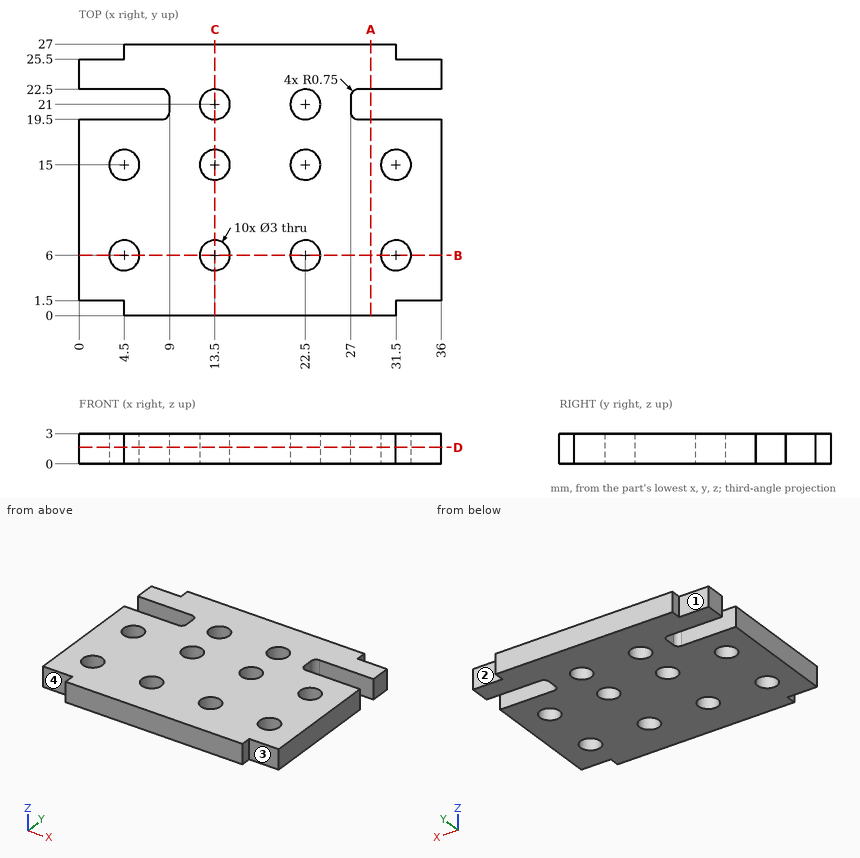
Could you check a few things on this drawing? It's one solid part, dimensions in mm from its lowest x, y, z. A direction names the side the tool comes from. Coordinates: 2 decimals unless noted, no trailing zeros. Order: outer loops, then holes, each group sorted by start corner. A loop starts at its lowest first (then second) coordinate and runs counter-clockwise, first axis right, second up. Notation, with made-up numbers: M 9.25,42 L 43.25,42 A22 ccw 43.25,48 Z; hole C 70,34 d6. An arc over 180 degrees is marked long. Use one line per item in the form item = value. Start each with the question number.
1. Suppose I cut it at A-A on x = 29. Write out the boundary of the cut face in (y, z), then the cut area to 3 significant figures.
2. Suppose I cut it at B-B on y = 6. Write out the boundary of the cut face in (x, z).
3. For pin 1 (1.5 mm diameter, centred on x = 3.5, z = 1, fed in from -Y); pin 2 (1.6 mm diameter, centred on y = 21, z = 1, fed in from -X); pin 3 (0.8 mm diameter, centred on y = 1, z = 2, fed in from -X); pin 4 (1.2 mm diameter, centred on y = 26, z = 1, fed in from -X), each with a flat end and sliding along its axis, tell me the tip position at first contact or that it passes through.
4. Suppose I cut it at D-D on z = 1.65. Count the separate pieces of the cut face and the enclosed holes in it, then the cut area to 3 significant figures.
5. Suppose I cut it at C-C on x = 13.5. Write out the boundary of the cut face in (y, z), then the cut area to 3 significant figures.
6. On a 3-axis mill with a long thin cutter (end or side, diameter ignored), from which of +Z, -Z, +X, -X, +Y, -Y can I reach the whole of each face in a straight line? I mean the marked faces 1, 2, 3 and 4. Say none if no direction works.
7. Please list where these lines run through material, in increasing order: line 1 (X direction, y = 6, z = 2.2); line 2 (Y direction, x = 13.5, z = 1.25); line 3 (X direction, y = 21, z = 2.2).
Geometry says:
q1.outline = M 0,0 L 19.5,0 L 19.5,3 L 0,3 Z; M 22.5,0 L 27,0 L 27,3 L 22.5,3 Z
q1.area = 72.0 mm^2
q2.outline = M 0,0 L 3,0 L 3,3 L 0,3 Z; M 6,0 L 12,0 L 12,3 L 6,3 Z; M 15,0 L 21,0 L 21,3 L 15,3 Z; M 24,0 L 30,0 L 30,3 L 24,3 Z; M 33,0 L 36,0 L 36,3 L 33,3 Z
q3.pin_1 = 1.5
q3.pin_2 = 9
q3.pin_3 = 4.5
q3.pin_4 = 0
q4.separate_pieces = 1
q4.enclosed_holes = 10
q4.area = 821 mm^2
q5.outline = M 0,0 L 4.5,0 L 4.5,3 L 0,3 Z; M 7.5,0 L 13.5,0 L 13.5,3 L 7.5,3 Z; M 16.5,0 L 19.5,0 L 19.5,3 L 16.5,3 Z; M 22.5,0 L 27,0 L 27,3 L 22.5,3 Z
q5.area = 54.0 mm^2
q6.face_1 = +Z, -Z, -X, +Y
q6.face_2 = +Z, -Z, +X, +Y
q6.face_3 = +Z, -Z, +X, -Y
q6.face_4 = +Z, -Z, -X, -Y
q7.line_1 = 0 to 3, 6 to 12, 15 to 21, 24 to 30, 33 to 36
q7.line_2 = 0 to 4.5, 7.5 to 13.5, 16.5 to 19.5, 22.5 to 27
q7.line_3 = 9 to 12, 15 to 21, 24 to 27
